from build123d import *

# Parameters (mm, degrees)
SKETCH1_W               = 48.3108
SKETCH1_H               = 30.03
BOSS_EXTRUDE1_DEPTH     = 2.95
SKETCH2_W               = 10.16
SKETCH2_H               = 12.7
CUT_EXTRUDE1_DEPTH      = 3.95
M3_CLEARANCE_HOLE1_D    = 3.2
SKETCH7_W               = 48.3108
SKETCH7_H               = 2.95
BOSS_EXTRUDE2_DEPTH     = 5
SKETCH6_W               = 10
SKETCH6_H               = 2.95
CUT_EXTRUDE2_DEPTH      = 3.95
LPATTERN1_COUNT         = 3
LPATTERN1_PITCH         = 20
MIRROR1_COPY_1_SKETCH_W = 10
MIRROR1_COPY_1_SKETCH_H = 2.95
MIRROR1_COPY_1_DEPTH    = 3.95
MIRROR1_COPY_2_SKETCH_W = 10
MIRROR1_COPY_2_SKETCH_H = 2.95
MIRROR1_COPY_2_DEPTH    = 3.95
SKETCH8_W               = 12.065
SKETCH8_H               = 2.95
BOSS_EXTRUDE3_DEPTH     = 7.9392
SKETCH9_W               = 17.065
SKETCH9_H               = 2.95
BOSS_EXTRUDE4_DEPTH     = 4.9892
SKETCH10_R              = 2.667
CUT_EXTRUDE3_DEPTH      = 3.95
SKETCH11_W              = 2.95
SKETCH11_H              = 10
CUT_EXTRUDE4_DEPTH      = 3.95


with BuildPart() as part:
    # Sketch1 → Boss-Extrude1 (new body)
    with BuildSketch(Plane(origin=(0, 0, 0), x_dir=(1, 0, 0), z_dir=(0, 1, 0))):
        Rectangle(SKETCH1_W, SKETCH1_H)
    extrude(amount=BOSS_EXTRUDE1_DEPTH)

    # Sketch2 → Cut-Extrude1 (cut, through all)
    with BuildSketch(Plane(origin=(0, 2.95, 0), x_dir=(1, 0, 0), z_dir=(0, 1, 0))):
        with Locations((-19.0754, 0)):
            Rectangle(SKETCH2_W, SKETCH2_H)
    extrude(amount=-CUT_EXTRUDE1_DEPTH, mode=Mode.SUBTRACT)

    # M3 Clearance Hole1 (through all)
    with Locations(Plane(origin=(0, 2.95, 0), x_dir=(1, 0, 0), z_dir=(0, 1, 0))):
        with Locations((-7.6454, 8.5725), (-7.6454, -8.5725)):
            Hole(M3_CLEARANCE_HOLE1_D / 2)

    # Sketch7 → Boss-Extrude2 (add)
    with BuildSketch(Plane.XY.offset(15.015)):
        with Locations((0, 1.475)):
            Rectangle(SKETCH7_W, SKETCH7_H)
    extrude(amount=BOSS_EXTRUDE2_DEPTH)

    # Sketch6 → Cut-Extrude2 (cut, through all)
    with BuildSketch(Plane(origin=(0, 2.95, 0), x_dir=(1, 0, 0), z_dir=(0, 1, 0))):
        with Locations((-19.1554, -18.54)):
            Rectangle(SKETCH6_W, SKETCH6_H)
    cut_extrude2 = extrude(amount=-CUT_EXTRUDE2_DEPTH, mode=Mode.SUBTRACT)

    # LPattern1: Cut-Extrude2 ×3
    with Locations(*[(i * LPATTERN1_PITCH, 0, 0) for i in range(1, LPATTERN1_COUNT)]):
        add(cut_extrude2, mode=Mode.SUBTRACT)

    # Mirror1: Cut-Extrude2 across plane
    add(cut_extrude2.mirror(Plane.XY.offset(2.5)), mode=Mode.SUBTRACT)

    # Mirror1 copy 1 sketch → Mirror1 copy 1 (cut, through all)
    with BuildSketch(Plane(origin=(20, 2.95, 5), x_dir=(1, 0, 0), z_dir=(0, 1, 0))):
        with Locations((-19.1554, 18.54)):
            Rectangle(MIRROR1_COPY_1_SKETCH_W, MIRROR1_COPY_1_SKETCH_H)
    extrude(amount=-MIRROR1_COPY_1_DEPTH, mode=Mode.SUBTRACT)

    # Mirror1 copy 2 sketch → Mirror1 copy 2 (cut, through all)
    with BuildSketch(Plane(origin=(40, 2.95, 5), x_dir=(1, 0, 0), z_dir=(0, 1, 0))):
        with Locations((-19.1554, 18.54)):
            Rectangle(MIRROR1_COPY_2_SKETCH_W, MIRROR1_COPY_2_SKETCH_H)
    extrude(amount=-MIRROR1_COPY_2_DEPTH, mode=Mode.SUBTRACT)

    # Sketch8 → Boss-Extrude3 (add)
    with BuildSketch(Plane(origin=(24.1554, 0, 0), x_dir=(0, 0, -1), z_dir=(1, 0, 0))):
        with Locations((6.0325, 1.475)):
            Rectangle(SKETCH8_W, SKETCH8_H)
    extrude(amount=BOSS_EXTRUDE3_DEPTH)

    # Sketch9 → Boss-Extrude4 (add)
    with BuildSketch(Plane(origin=(24.1554, 0, 0), x_dir=(0, 0, -1), z_dir=(1, 0, 0))):
        with Locations((-8.5325, 1.475)):
            Rectangle(SKETCH9_W, SKETCH9_H)
    extrude(amount=BOSS_EXTRUDE4_DEPTH)

    # Sketch10 → Cut-Extrude3 (cut, through all)
    with BuildSketch(Plane.XZ):
        with Locations((12.827, 0)):
            Circle(SKETCH10_R)
    extrude(amount=-CUT_EXTRUDE3_DEPTH, mode=Mode.SUBTRACT)

    # Sketch11 → Cut-Extrude4 (cut, through all)
    with BuildSketch(Plane.XZ):
        with Locations((4.3696, -7.065)):
            Rectangle(SKETCH11_W, SKETCH11_H)
    extrude(amount=-CUT_EXTRUDE4_DEPTH, mode=Mode.SUBTRACT)


solid = part.part
Source: CAD feature listing. Evaluate the final solid. Frame: model axes, mm. A direction names the side the tool comes from. Give positions to 0.01 mm unless a question says otherwise; leave off trailing zeros. Loops run counter-clockwise (first coordinate to the right, second up) from the corner with the lowest first, then second, coordinate; pieces in that order, holes last. Notation, with made-up numbers: (72.5, 59) -> (106.5, 59) arc R14 cw to (106.5, 81) -> close; hole circle Ø10 at (54, 41). An arc over 180 degrees is marked (long way). Use a Markdown table: item, result. Add a question column.
1) Section query D-D, the plane x = 24. Return the cut outline in (y, z) (3 decimals), then the cut area to 3 significant figures.
2) First-contact query: pin 1 (1.5 mm diameter, centred on y = 1.5, z = 19, fed in from +X); pin 2 (0.9 mm diameter, centred on x = -0.5, y = 1, fed in from -Z) (3 decimals); pin 3 (0.9 mm diameter, centred on y = 1, z = 18, fed in from -X); pin 4 (1 mm diameter, centred on x = 22.5, z = -9, fed in from -Y). Flat tips, straight axial feed; report the tip coordinate or a pass-through.
3) Section query A-A, the plane z = -4. Return the cut outline in (x, y).
4) Section query B-B, the plane x = 11. Return the cut outline in (y, z) (3 decimals), then the cut area to 3 significant figures.
5) Line query: line 1 along X through (y, z) = (1.25, 17.5); line 2 along X through (y, z) = (1.2, -9.5); line 3 along X through (y, z) = (1.95, -8). Output: solid intervals per line, ascending. Write a range as [from, to].
6) Section query C-C, the plane y = 0.45. Count the separate pieces of the cut face and the enclosed holes in it, then the cut area to 3 significant figures.
7) Pull-direction query (Z, two-part tool) for faces 1 (the face through (-9, 1, -15.015)), 2 (the face through (-9, 1, 20.015)), 3 (the face through (-19, 1, 6.35)), 4 (the face through (29.145, 1, 9)); classes: +Z half, -Z half, draft (parallel to the pull), parting line (faces both ways), or undercut.
8) Reachability of faces 5 (the face through (1, 1, 17.065)), 6 (the face through (15.845, 1, 19)), 7 (the face through (-13.995, 1, 0)) from +Z, -Z, +X, -X, +Y, -Y: full face, straight path, thin tool, end or side. Return the list, or none.
Numbers:
| question | item | result |
|---|---|---|
| 1 | outline | (0, -12.065) -> (2.95, -12.065) -> (2.95, 17.065) -> (0, 17.065) -> close |
| 1 | area | 85.9 mm2 |
| 2 | pin 1 | stops at x = 15.84 |
| 2 | pin 2 | stops at z = -12.065 |
| 2 | pin 3 | stops at x = -14.16 |
| 2 | pin 4 | stops at y = 0 |
| 3 | outline | (-14, 0) -> (2.89, 0) -> (2.89, 2.95) -> (-14, 2.95) -> close; (5.84, 0) -> (32.09, 0) -> (32.09, 2.95) -> (5.84, 2.95) -> close |
| 4 | outline | (0, -15.015) -> (2.95, -15.015) -> (2.95, -1.943) -> (0, -1.943) -> close; (0, 1.943) -> (2.95, 1.943) -> (2.95, 20.015) -> (0, 20.015) -> close |
| 4 | area | 91.9 mm2 |
| 5 | line 1 | x = [-14.16, -4.16], [5.84, 15.84] |
| 5 | line 2 | x = [-24.16, -8.95], [-6.34, 2.89], [5.84, 32.09] |
| 5 | line 3 | x = [-24.16, -9.14], [-6.15, 2.89], [5.84, 32.09] |
| 6 | separate pieces | 1 |
| 6 | enclosed holes | 3 |
| 6 | area | 1,510 mm2 |
| 7 | face 1 | -Z half |
| 7 | face 2 | +Z half |
| 7 | face 3 | undercut |
| 7 | face 4 | draft |
| 8 | face 5 | +Z, +Y, -Y |
| 8 | face 6 | +Z, +X, +Y, -Y |
| 8 | face 7 | -X, +Y, -Y |
